```python
from build123d import *

# Parameters (mm, degrees)
BOSS_EXTRUDE1_DEPTH = 50
SKETCH2_W           = 11
SKETCH2_H           = 20
BOSS_EXTRUDE2_DEPTH = 30
CUT_EXTRUDE1_DEPTH  = 65.567793829
SKETCH4_R           = 1.75
CUT_EXTRUDE2_DEPTH  = 30
SKETCH5_R           = 2
CUT_EXTRUDE3_DEPTH  = 30
SKETCH6_W           = 11
SKETCH6_H           = 5.5
CUT_EXTRUDE4_DEPTH  = 2


with BuildPart() as part:
    # Sketch1 → Boss-Extrude1 (new body)
    with BuildSketch(Plane.XY):
        Polygon((0, 38), (0, 0), (15, 0), (15, 3), (4, 3), (4, 38), align=None)
    extrude(amount=BOSS_EXTRUDE1_DEPTH)

    # Sketch2 → Boss-Extrude2 (add)
    with BuildSketch(Plane(origin=(0, 3, 0), x_dir=(1, 0, 0), z_dir=(0, 1, 0))):
        with Locations((9.5, -25)):
            Rectangle(SKETCH2_W, SKETCH2_H)
    extrude(amount=BOSS_EXTRUDE2_DEPTH)

    # Sketch3 → Cut-Extrude1 (cut, through all)
    with BuildSketch(Plane.XY.offset(50)):
        Polygon((4, 33), (4, 17), (15, 3), (15, 33), align=None)
    extrude(amount=-CUT_EXTRUDE1_DEPTH, mode=Mode.SUBTRACT)

    # Sketch4 → Cut-Extrude2 (cut)
    with BuildSketch(Plane.ZY):
        with Locations(Location((5.1, 11.6, 0), (0, 0, 270))):
            Circle(SKETCH4_R)
        with Locations(Location((11.6, 30.5, 0), (0, 0, 270))):
            Circle(SKETCH4_R)
        with Locations(Location((45.1, 11.6, 0), (0, 0, 270))):
            Circle(SKETCH4_R)
        with Locations(Location((38.6, 30.5, 0), (0, 0, 270))):
            Circle(SKETCH4_R)
    extrude(amount=-CUT_EXTRUDE2_DEPTH, mode=Mode.SUBTRACT)

    # Sketch5 → Cut-Extrude3 (cut)
    with BuildSketch(Plane(origin=(0, 3, 0), x_dir=(1, 0, 0), z_dir=(0, 1, 0))):
        with Locations(Location((9.5, -43, 0), (0, 0, 270))):
            Circle(SKETCH5_R)
        with Locations(Location((9.5, -7, 0), (0, 0, 180))):
            Circle(SKETCH5_R)
    extrude(amount=-CUT_EXTRUDE3_DEPTH, mode=Mode.SUBTRACT)

    # Sketch6 → Cut-Extrude4 (cut)
    with BuildSketch(Plane.ZY):
        with Locations((34.35, 11.25)):
            Rectangle(SKETCH6_W, SKETCH6_H)
    extrude(amount=-CUT_EXTRUDE4_DEPTH, mode=Mode.SUBTRACT)


solid = part.part
```
Here's how the part is built. I have some questions about the finished solid (model axes, mm). A direction names the side the tool comes from. Round coordinates to 2 decimals unless told otherwise and drop trailing zeros. Order: outer loops, then holes, each group sorted by start corner. A loop starts at its lowest first (then second) coordinate and runs counter-clockwise, first axis right, second up. Notation, with made-up numbers: M 27,-3.75 L 34,-3.75 A19 ccw 34,9.25 Z; hole C 64.5,11.5 d1. An arc over 180 degrees is marked long. Answer as CSV lines item,"result".
Item 1: Imagine slicing it at A-A on y = 30.5. List the corners of the cut face in (x, z) for me.
From the geometry:
outline,"M 0,0 L 4,0 L 4,9.85 L 0,9.85 Z; M 0,13.35 L 4,13.35 L 4,36.85 L 0,36.85 Z; M 0,40.35 L 4,40.35 L 4,50 L 0,50 Z"
Item 2: Which directions (+Z, -Z, +X, -X, +Y, -Y) give clear straight access to the entire face, cutting with the end or side of a thin tool? Please do faces 1 (the flat face through (4, 20, 25)), 2 (the flat face through (8, 8, 35)), 3 (the flat face through (1, 11, 39.85)).
From the geometry:
face 1,"+X, +Y"
face 2,"+Z, +X, +Y"
face 3,"-X"
Item 3: For pin 1 (5.5 mm diameter, centred on x = 8.5, z = 39, fed in from +Y); pin 2 (2 mm diameter, centred on x = 11, y = 8, fed in from +Z); pin 3 (3.5 mm diameter, centred on x = 12, y = 8.5, fed in from -Z), each with a flat end and sliding along its axis, tell me the tip position at first contact or that it passes through.
From the geometry:
pin 1,"y = 3"
pin 2,"z = 35"
pin 3,"z = 15"
Item 4: Please list where these lines run through material, in increasing order: L1, parallel to Z at x = 2.3, y = 30.5; L2, parallel to Z at x = 0.8, y = 11.6; L3, parallel to Y at x = 1.25, z = 33.5. Write a range as [from, to].
From the geometry:
L1,"[0, 9.85], [13.35, 36.85], [40.35, 50]"
L2,"[0, 3.35], [6.85, 28.85], [39.85, 43.35], [46.85, 50]"
L3,"[0, 8.5], [14, 38]"
Item 5: We'd pull the mould along Y, two halves only. Please class faces 4 (the cylindrical face through (2, 10.7, 6.6)), 5 (the flat face through (11, 3, 9)), 6 (the flat face through (8, 8, 15)): +Y half, -Y half, draft (parallel to the pull), parting line (faces both ways), or undercut.
From the geometry:
face 4,"undercut"
face 5,"+Y half"
face 6,"draft"
Item 6: Imagine slicing it at D-D on z = 19.5. List the corners of the cut face in (x, y) for me, and give its area (3 significant figures).
From the geometry:
outline,"M 0,0 L 15,0 L 15,3 L 4,17 L 4,38 L 0,38 Z"
area,"262 mm2"
Item 7: Imagine slicing it at B-B on x = 9.5. List the corners of the cut face in (y, z) for me, and give its area (3 significant figures).
From the geometry:
outline,"M 0,0 L 3,0 L 3,5 L 0,5 Z; M 0,9 L 3,9 L 3,15 L 10,15 L 10,35 L 3,35 L 3,41 L 0,41 Z; M 0,45 L 3,45 L 3,50 L 0,50 Z"
area,"266 mm2"
Item 8: Imagine slicing it at C-C on z = 38.6. List the corners of the cut face in (x, y) for me.
From the geometry:
outline,"M 0,0 L 15,0 L 15,3 L 4,3 L 4,28.75 L 0,28.75 L 0,14 L 2,14 L 2,8.5 L 0,8.5 Z; M 0,32.25 L 4,32.25 L 4,38 L 0,38 Z"
